The listing builds one solid part. Answer for the finished solid, in the listing's coordinates (mm). Face numbers are marked on the shaded views. A direction names the side the tool comes from. Coordinates: 2 decimals unless noted, no trailing zeros. Order: outer loops, then holes, each group sorted by start corner. A loop starts at its lowest first (then second) coordinate and runs counter-clockwise, first axis right, second up. Notation, with made-up numbers: M 18.25,54.25 L 32.25,54.25 A24 ccw 32.25,72.25 Z; hole C 11,21.5 d2. An arc over 180 degrees is marked long. One line per item, written item: value. Start each with the question number.
Q1. The part is cut by section B-B on x = 16. Give the vertices of the cut face in (y, z).
Q2. The part is cut by section C-C on x = -8.5. Give the vertices of the cut face in (y, z), then the cut area to 3 significant figures.
Q3. For the marked faces 1, 2 and 3, determine the directions among +Z, -Z, +X, -X, +Y, -Y from which every point of the face is accessible in a straight line to the end or side of a thin tool.
Q4. The part is cut by section A-A on z = -27.5. Give the vertices of the cut face in (x, y).
Q5. The part is cut by section D-D on x = 0. Give the vertices of the cut face in (y, z).
Q6. Straight lines are drawn through the part: line 1 along Y through (x, z) = (0, -0.6); line 2 along Y through (x, z) = (-21.9, -27.5); line 3 along Y through (x, z) = (16, 0.95). For each, find the intervals that lie inside material, in ascending order. Write a range as [from, to].
Q7. Each of these flat-tipped pins is pushed along its axis until it touches: pin 1 Ø6 at (y, z) = (2.5, -30) entering from +X; pin 2 Ø1 at (x, z) = (-7, -17) entering from +Y; pin 3 Ø6.5 at (x, y) = (16, 1.5) entering from +Z; pin 4 Ø8 at (x, y) = (17, -47) entering from -Z. Where does it stop, or does it pass through?
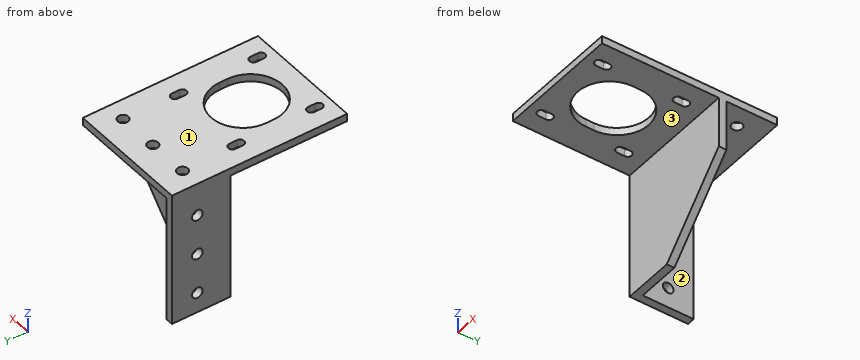
Autodesk Inventor part; units mm, degrees
ref_plane "YZ Plane" through (0, 0, 0) normal (1, 0, 0) x (0, 1, 0)
ref_plane "XZ Plane" through (0, 0, 0) normal (0, 1, 0) x (-1, 0, 0)
ref_plane "XY Plane" through (0, 0, 0) normal (0, 0, 1) x (1, 0, 0)
sketch "Sketch1" plane through (0, 0, 0) normal (0, 0, 1) x (1, 0, 0)
  line L0 (-24, 11.5) -> (-24, -11.5)
  line L1 (-24, -11.5) -> (24, -11.5) construction
  line L2 (24, -11.5) -> (24, 11.5)
  line L3 (24, 11.5) -> (-1, 11.5)
  line L4 (-1, 11.5) -> (-24, 11.5)
  line L5 (-24, -11.5) -> (-24, -57.5)
  line L6 (-24, -57.5) -> (24, -57.5)
  line L7 (24, -57.5) -> (24, -11.5)
  point P0 (0, 0)
  point P1 (0, -11.5)
  point P2 (-24, 0)
  point P3 (11.5, 11.5)
  dimension "d0" = 23
  dimension "d1" = 23
  dimension "d2" = 48
  dimension "d6" = 48
  dimension "d7" = 46
extrude "Extrusion1" add sketch "Sketch1" along normal mid plane 3
sketch "Sketch2" plane through (0, 0, 1.5) normal (0, 0, 1) x (1, 0, 0)
  arc A0 (-17.1, -52.5) -> (-13.9, -52.5) centre (-15.5, -52.5) ccw
  arc A1 (-13.9, -18.5) -> (-17.1, -18.5) centre (-15.5, -18.5) ccw
  arc A2 (17.1, -18.5) -> (13.9, -18.5) centre (15.5, -18.5) ccw
  arc A3 (13.9, -52.5) -> (17.1, -52.5) centre (15.5, -52.5) ccw
  arc A4 (-17.1, -21.5) -> (-13.9, -21.5) centre (-15.5, -21.5) ccw
  arc A5 (-13.9, -49.5) -> (-17.1, -49.5) centre (-15.5, -49.5) ccw
  arc A6 (13.9, -21.5) -> (17.1, -21.5) centre (15.5, -21.5) ccw
  arc A7 (17.1, -49.5) -> (13.9, -49.5) centre (15.5, -49.5) ccw
  line L0 (-17.1, -52.5) -> (-17.1, -49.5)
  line L1 (-13.9, -52.5) -> (-13.9, -49.5)
  line L2 (-17.1, -21.5) -> (-17.1, -18.5)
  line L3 (-13.9, -18.5) -> (-13.9, -21.5)
  line L4 (13.9, -18.5) -> (13.9, -21.5)
  line L5 (17.1, -21.5) -> (17.1, -18.5)
  line L6 (13.9, -49.5) -> (13.9, -52.5)
  line L7 (17.1, -52.5) -> (17.1, -49.5)
  line L8 (-24, 11.5) -> (-24, -57.5)
  line L9 (-24, -57.5) -> (24, -57.5)
  line L10 (-17.1, -51) -> (-13.9, -51) construction
  line L11 (-17.1, -20) -> (-13.9, -20) construction
  point P0 (0, 0)
  dimension "d8" = 3.2
  dimension "d9" = 3
  dimension "d10" = 8.5
  dimension "d11" = 5
  dimension "d12" = 31
  dimension "d13" = 31
  dimension "d14" = 3
extrude "Extrusion2" cut sketch "Sketch2" against normal up to next
sketch "Sketch3" plane through (0, 0, 1.5) normal (0, 0, 1) x (1, 0, 0)
  line L0 (24, 11.5) -> (24, -57.5)
  line L1 (24, 11.5) -> (-24, 11.5) construction
  line L2 (-24, -57.5) -> (-24, 11.5)
  line L3 (24, 11.5) -> (24, -57.5)
  line L4 (24, -57.5) -> (24, 11.5)
  line L5 (-24, 11.5) -> (24, 11.5)
  circle A0 centre (16, 1.5) radius 2.1
  circle A1 centre (0, 1.5) radius 2.1
  circle A2 centre (-16, 1.5) radius 2.1
  point P0 (0, 0)
  point P1 (35, -11.5)
  point P2 (16.6018, 1.5)
  dimension "d19" = 4.2
  dimension "d20" = 16
  dimension "d21" = 8
  dimension "d23" = 16
  dimension "d52" = 10
sketch "Sketch4" plane through (0, 0, -1.5) normal (0, 0, -1) x (-1, 0, 0)
  line L0 (13.9, -21.5) -> (13.9, -18.5)
  arc A0 (17.1, -18.5) -> (13.9, -18.5) centre (15.5, -18.5) ccw
  line L1 (17.1, -18.5) -> (17.1, -21.5)
  arc A1 (13.9, -21.5) -> (17.1, -21.5) centre (15.5, -21.5) ccw
  arc A2 (13.9, -52.5) -> (17.1, -52.5) centre (15.5, -52.5) ccw
  line L2 (13.9, -52.5) -> (13.9, -49.5)
  arc A3 (17.1, -49.5) -> (13.9, -49.5) centre (15.5, -49.5) ccw
  line L3 (17.1, -49.5) -> (17.1, -52.5)
  line L4 (-17.1, -52.5) -> (-17.1, -49.5)
  arc A4 (-13.9, -49.5) -> (-17.1, -49.5) centre (-15.5, -49.5) ccw
  line L5 (-13.9, -49.5) -> (-13.9, -52.5)
  arc A5 (-17.1, -52.5) -> (-13.9, -52.5) centre (-15.5, -52.5) ccw
  line L6 (-17.1, -21.5) -> (-17.1, -18.5)
  arc A6 (-13.9, -18.5) -> (-17.1, -18.5) centre (-15.5, -18.5) ccw
  line L7 (-13.9, -18.5) -> (-13.9, -21.5)
  arc A7 (-17.1, -21.5) -> (-13.9, -21.5) centre (-15.5, -21.5) ccw
  line L8 (24, -57.5) -> (24, 11.5)
  line L9 (24, 11.5) -> (-24, 11.5)
  line L10 (-24, 11.5) -> (-24, -57.5)
  line L11 (-24, -57.5) -> (24, -57.5)
  line L12 (-24, 11.5) -> (-24, -11.5)
  line L13 (-24, -11.5) -> (24, -11.5)
  line L14 (24, -57.5) -> (24, 11.5)
  line L15 (24, -8.5) -> (-24, -8.5)
  point P0 (0, 0)
  point P1 (-35, -11.5)
  dimension "d30" = 3
extrude "Extrusion4" add sketch "Sketch4" along normal blind 50 contours L13 L10 L15 L8
sketch "Sketch8" plane through (0, 0, 1.5) normal (0, 0, 1) x (1, 0, 0)
  arc A0 (12.5, -34) -> (-12.5, -34) centre (0, -34) ccw
  arc A1 (-12.5, -37) -> (12.5, -37) centre (0, -37) ccw
  line L0 (13.9, -21.5) -> (13.9, -18.5)
  line L1 (13.9, -20) -> (-13.9, -20) construction
  line L2 (-13.9, -18.5) -> (-13.9, -21.5)
  line L3 (-13.9, -20) -> (-13.9, -51) construction
  line L4 (-13.9, -49.5) -> (-13.9, -52.5)
  line L5 (12.5, -34) -> (12.5, -37)
  line L6 (-12.5, -34) -> (-12.5, -37)
  point P0 (0, 0)
  point P1 (-12.5, -35.5)
  point P2 (-13.9, -35.5)
  point P3 (0, -21.5)
  point P4 (0, -20)
  dimension "d46" = 25
  dimension "d47" = 3
extrude "Extrusion8" cut sketch "Sketch8" against normal up to next
sketch "Sketch9" plane through (-24, -57.5, 1.5) normal (-1, 0, 0) x (0, 0, 1)
  line L0 (-3, 69) -> (-3, 49)
  line L1 (-3, 69) -> (-53, 69)
  line L2 (-3, 49) -> (-53, 49)
  line L3 (-53, 46) -> (-53, 49)
  line L4 (-53, 69) -> (-53, 49)
  point P0 (-1.5, 57.5)
  point P1 (-53, 0)
extrude "Extrusion9" add sketch "Sketch9" against normal blind 3
extrude "Extrusion10" cut sketch "Sketch3" against normal up to next
sketch "Sketch10" plane through (-24, -11.5, -1.5) normal (0, -1, 0) x (1, 0, 0)
  line L0 (48, 0) -> (48, -50)
  line L1 (48, -20) -> (20, -50)
  line L2 (48, 0) -> (0, 0)
  line L3 (0, 0) -> (0, -50)
  line L4 (48, -50) -> (0, -50)
  point P0 (24, 1.5)
  dimension "d55" = 20
  dimension "d56" = 20
extrude "Extrusion11" cut sketch "Sketch10" against normal up to next contours L0 L4 L1
sketch "Sketch11" plane through (-24, -57.5, 1.5) normal (-1, 0, 0) x (0, 0, 1)
  circle A0 centre (-13, 59) radius 2.1
  circle A1 centre (-45, 59) radius 2.1
  circle A2 centre (-29, 59) radius 2.1
  line L0 (0, 69) -> (0, 0)
  line L1 (0, 69) -> (-53, 69)
  point P0 (-1.5, 57.5)
  dimension "d59" = 4.2
  dimension "d60" = 16
  dimension "d61" = 13
  dimension "d62" = 16
  dimension "d65" = 10
extrude "Extrusion12" cut sketch "Sketch11" against normal up to next
properties part number "MotorMount2"
Output:
1. outline: M -57.5,-1.5 L -54.02,-1.5 L -54.02,1.5 L -57.5,1.5 Z; M -47.98,-1.5 L -23.02,-1.5 L -23.02,1.5 L -47.98,1.5 Z; M -16.98,-1.5 L -11.5,-1.5 L -11.5,-30.07 L -8.5,-30.07 L -8.5,-1.5 L -0.6,-1.5 L -0.6,1.5 L -16.98,1.5 Z; M 3.6,-1.5 L 11.5,-1.5 L 11.5,1.5 L 3.6,1.5 Z
2. outline: M -57.5,-1.5 L -46.17,-1.5 L -46.17,1.5 L -57.5,1.5 Z; M -24.83,-1.5 L -11.5,-1.5 L -11.5,-51.5 L -8.5,-51.5 L -8.5,-1.5 L 11.5,-1.5 L 11.5,1.5 L -24.83,1.5 Z
2. area: 293 mm^2
3. face 1: +Z, +X, -X, +Y, -Y
3. face 2: -Z, +X, +Y
3. face 3: -Z, +X, -X, -Y
4. outline: M -24,-11.5 L 18.4,-11.5 L 18.4,-8.5 L -21,-8.5 L -21,-0.6 L -24,-0.6 Z; M -24,3.6 L -21,3.6 L -21,11.5 L -24,11.5 Z
5. outline: M -57.5,-1.5 L -49.5,-1.5 L -49.5,1.5 L -57.5,1.5 Z; M -21.5,-1.5 L -11.5,-1.5 L -11.5,-47.21 L -8.5,-47.21 L -8.5,-1.5 L -0.6,-1.5 L -0.6,1.5 L -21.5,1.5 Z; M 3.6,-1.5 L 11.5,-1.5 L 11.5,1.5 L 3.6,1.5 Z
6. line 1: y = [-57.5, -49.5], [-21.5, -0.6], [3.6, 11.5]
6. line 2: y = [-11.5, -0.6], [3.6, 11.5]
6. line 3: y = [-57.5, -54.02], [-47.98, -23.02], [-16.98, -0.6], [3.6, 11.5]
7. pin 1: stops at x = -21
7. pin 2: stops at y = -8.5
7. pin 3: stops at z = 1.5
7. pin 4: stops at z = -1.5
